Source: three-view drawing plus pictorial views. Frame: mm from the lowest corner of the part. Round coordinates to 2 decimals unless told otherwise and drop trailing zeros. Loops run counter-clockwise (first coordinate to the right, second up) from the corner with the lowest first, then second, coordinate; pieces in that order, holes last. Notation, with made-up numbers: M 18.5,64 L 52.5,64 A18 cw 52.5,91 Z; hole C 66,87 d11. An arc over 180 degrees is marked long. Write each question's results on one line, items separated by ' | '.
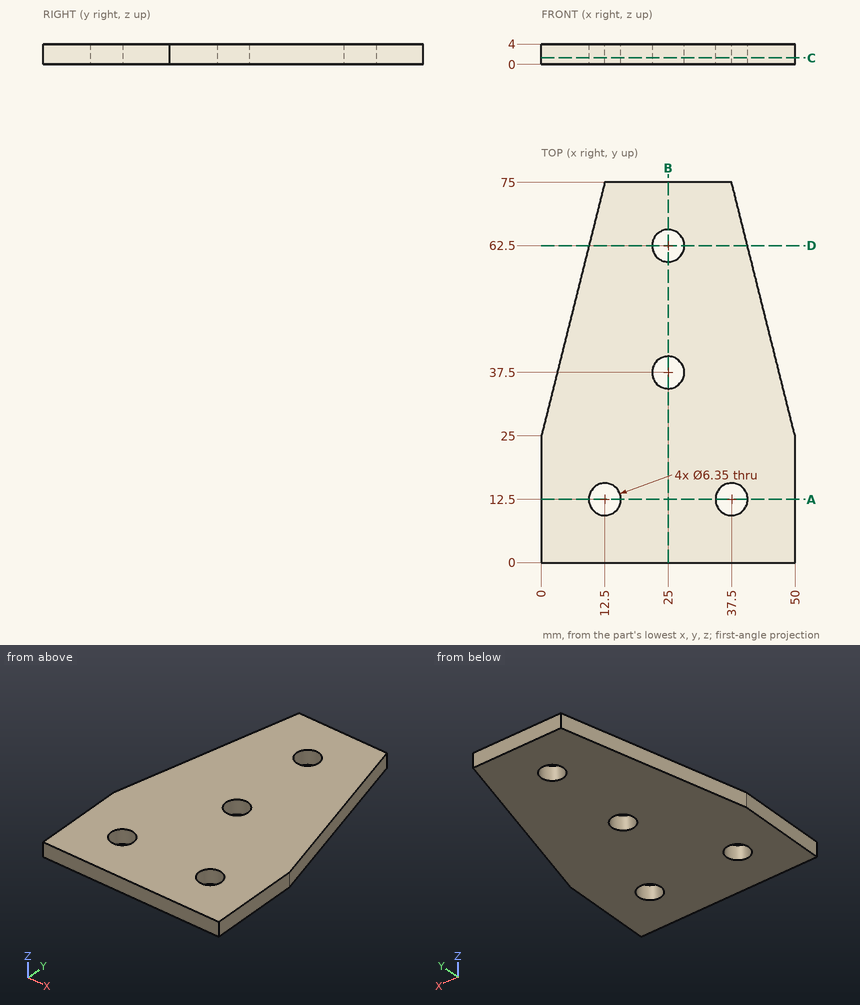
1. Pin query (flat end, axial travel): P1, Ø1, axis at y = 37, z = 2, coming from the -X side (3 decimals); P2, Ø2, axis at y = 29.5, z = 3, coming from the +X side (3 decimals). Return the tip coordinate at first contact, or that it passes through.
Answer key:
P1: stops at x = 2.875 | P2: stops at x = 49.125
2. Section A-A (y = 12.5). Output: boundary loops of the cut face in (x, z) (3 decimals).
Answer key:
outline: M 0,0 L 9.325,0 L 9.325,4 L 0,4 Z; M 15.675,0 L 34.325,0 L 34.325,4 L 15.675,4 Z; M 40.675,0 L 50,0 L 50,4 L 40.675,4 Z
3. Section D-D (y = 62.5). Output: boundary loops of the cut face in (x, z) (3 decimals), then the cut area to 3 significant figures.
Answer key:
outline: M 9.375,0 L 21.825,0 L 21.825,4 L 9.375,4 Z; M 28.175,0 L 40.625,0 L 40.625,4 L 28.175,4 Z | area: 99.6 mm²
4. Section C-C (z = 1.25). Output: boundary loops of the cut face in (x, y) (3 decimals), then the cut area to 3 significant figures.
Answer key:
outline: M 0,0 L 50,0 L 50,25 L 37.5,75 L 12.5,75 L 0,25 Z; hole C 12.5,12.5 d6.35; hole C 25,37.5 d6.35; hole C 25,62.5 d6.35; hole C 37.5,12.5 d6.35 | area: 3,000 mm²
5. Ray query, probe 1 along Y at (x, z) = (25, 1.2) (3 decimals); probe 2 along X at (y, z) = (12, 2.1); probe 3 along X at (y, z) = (38.5, 2.75) (3 decimals). Return the intervals inside material, ascending.
Answer key:
probe 1: y = 0 to 34.325, 40.675 to 59.325, 65.675 to 75 | probe 2: x = 0 to 9.36, 15.64 to 34.36, 40.64 to 50 | probe 3: x = 3.375 to 21.987, 28.013 to 46.625
6. Section B-B (x = 25). Output: boundary loops of the cut face in (y, z) (3 decimals).
Answer key:
outline: M 0,0 L 34.325,0 L 34.325,4 L 0,4 Z; M 40.675,0 L 59.325,0 L 59.325,4 L 40.675,4 Z; M 65.675,0 L 75,0 L 75,4 L 65.675,4 Z
